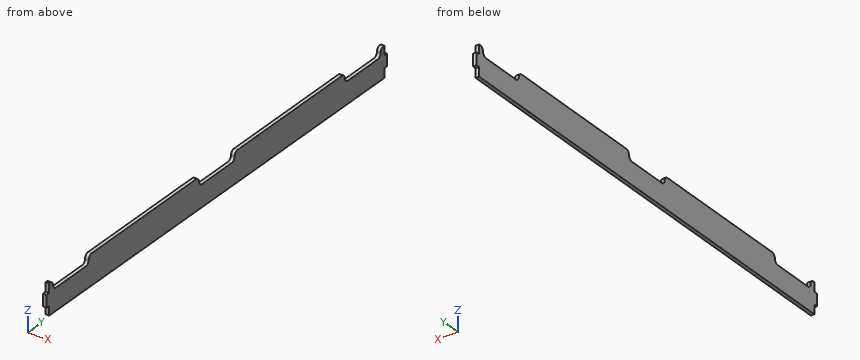
```python
from build123d import *

# Parameters (mm, degrees)
PAD002_DEPTH        = 3
POCKET_DEPTH        = 3
LINEARPATTERN_COUNT = 3
LINEARPATTERN_PITCH = 171.5


with BuildPart() as part:
    # Sketch002 → Pad002 (new body)
    with BuildSketch(Plane.YZ):
        Polygon((0, -17.5), (394, -17.5), (394, -10), (397, -10), (397, 0), (394, 0), (394, 7.5), (0, 7.5), (0, 0), (-3, 0), (-3, -10), (0, -10), align=None)
    extrude(amount=PAD002_DEPTH)

    # Sketch003 → Pocket (cut)
    with BuildSketch(Plane.YZ.offset(3)):
        with BuildLine():
            ThreePointArc((4.499999, 4.000001), (5.525124, 1.525129), (7.999997, 0.500003))
            Line((7.999997, 0.500003), (42.999997, 0.500003))
            ThreePointArc((42.999997, 0.500003), (45.474872, 1.525128), (46.499999, 4.000001))
            ThreePointArc((49.999997, 7.5), (47.525124, 6.474874), (46.499999, 4.000001))
            Line((1, 7.5), (49.999997, 7.5))
            ThreePointArc((4.499999, 4.000001), (3.474873, 6.474874), (1, 7.5))
        make_face()
    pocket = extrude(amount=-POCKET_DEPTH, mode=Mode.SUBTRACT)

    # LinearPattern: Pocket ×3
    with Locations(*[(0, i * LINEARPATTERN_PITCH, 0) for i in range(1, LINEARPATTERN_COUNT)]):
        add(pocket, mode=Mode.SUBTRACT)


with BuildPart() as part_1:
    # Body002 placement: moved
    add(part.part.moved(Location((91, 0, 31))))


solid = part_1.part
```
Here's how the part is built. I have some questions about the finished solid (model axes, mm). Give positions to 0.01 mm unless a question says otherwise; leave off trailing zeros. Order: outer loops, then holes, each group sorted by start corner. A loop starts at its lowest first (then second) coordinate and runs counter-clockwise, first axis right, second up. Notation, with made-up numbers: M 87,-27 L 146,-27 A34 ccw 146,8 Z; hole C 88,1 d10. An arc over 180 degrees is marked long. Use a Markdown table: item, result. Add a question column.
1. For pin 1 Ø0.9 at (x, y) = (93, -1.5) entering from -Z; pin 2 Ø0.9 at (x, y) = (93, -1) entering from +Z; pin 3 Ø1.5 at (x, y) = (92, 18.5) entering from +Z, each with a flat end and sliding along its axis, tell me the tip position at first contact or that it passes through.
2. Suppose I cut it at B-B (y = 183). List the corners of the cut face in (x, z) for me.
3. I need wall thicknesses on probe 1 along Y at (x, z) = (91.5, 35.5); probe 2 along Y at (x, z) = (92.2, 32.5); probe 3 along Y at (x, z) = (91.85, 20.75). Which ranges of each line are inside material? Lowest first, please. Write a range as from..to.
Results list:
| question | item | result |
|---|---|---|
| 1 | pin 1 | stops at z = 21 |
| 1 | pin 2 | stops at z = 31 |
| 1 | pin 3 | stops at z = 31.5 |
| 2 | outline | M 91,13.5 L 94,13.5 L 94,31.5 L 91,31.5 Z |
| 3 | probe 1 | y = 0..4.46, 46.54..175.96, 218.04..347.46, 389.54..394 |
| 3 | probe 2 | y = 0..5.55, 45.45..177.05, 216.95..348.55, 388.45..394 |
| 3 | probe 3 | y = 0..394 |
